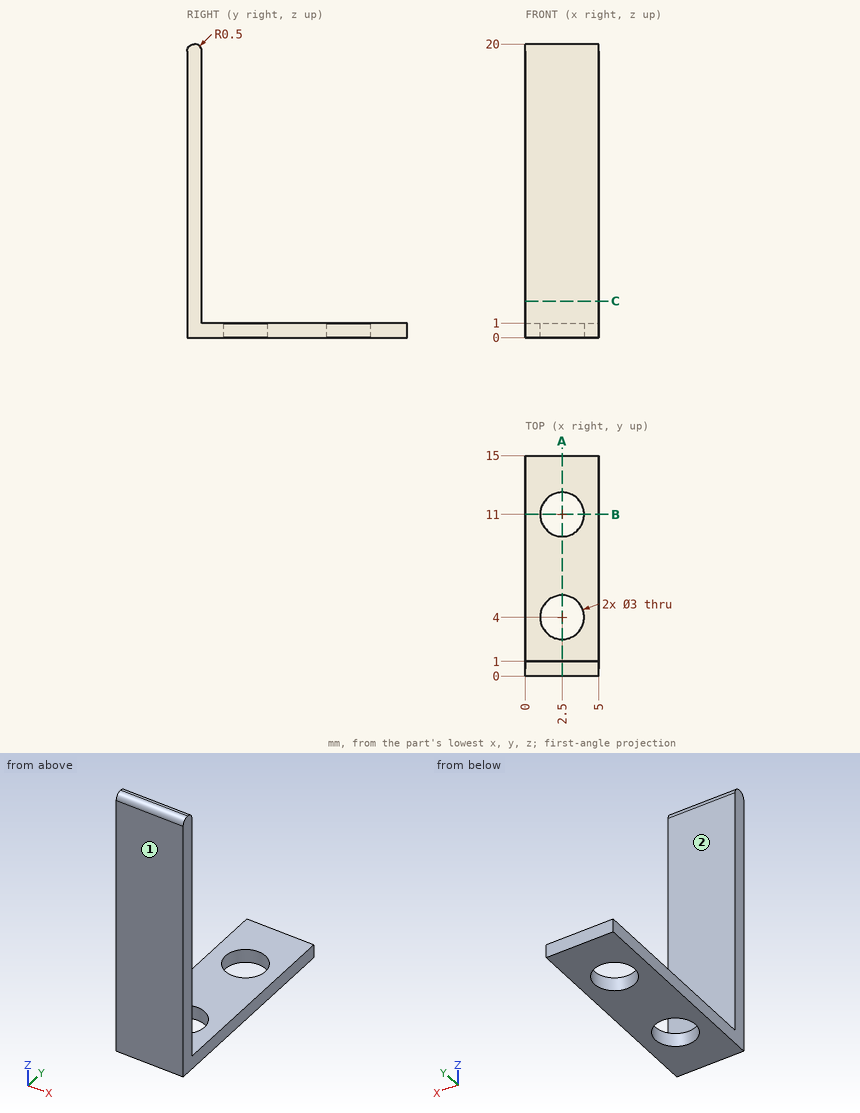
Answer from the drawing. Dimensions are ordinates in mm from the lowest x, y and z of the part. A direction names the side the tool comes from. Round coordinates to 2 decimals unless told otherwise and drop trailing zeros. Loops run counter-clockwise (first coordinate to the right, second up) from the corner with the lowest first, then second, coordinate; pieces in that order, holes last. Notation, with made-up numbers: (41.25, 84) - (99.25, 84) arc R27 cw to (99.25, 119) - close; hole circle Ø10 at (-8.75, -33.75). An arc over 180 degrees is marked (long way). One line per item, written item: value.
Q1. Find section A-A on x = 2.5. State how many separate pieces and enclosed holes the cut face has, and give its area (3 significant figures).
Check values:
separate pieces: 3
enclosed holes: 0
area: 27.9 mm2
Q2. Straight lines are drawn through the part: probe 1 along Y at (x, z) = (2.5, 0.25); probe 2 along Z at (x, y) = (1.45, 13.75). For each, find the intervals that lie inside material, in ascending order.
Check values:
probe 1: 0 to 2.5, 5.5 to 9.5, 12.5 to 15
probe 2: 0 to 1
Q3. Find section B-B on y = 11. Give the vertices of the cut face in (x, z), and give its area (3 significant figures).
Check values:
outline: (0, 0) - (1, 0) - (1, 1) - (0, 1) - close; (4, 0) - (5, 0) - (5, 1) - (4, 1) - close
area: 2.00 mm2
Q4. Find section C-C on z = 2.5. Give the vertices of the cut face in (x, y).
Check values:
outline: (0, 0) - (5, 0) - (5, 1) - (0, 1) - close
Q5. For the marked faces 1 and 2, determine the directions among +Z, -Z, +X, -X, +Y, -Y from which every point of the face is accessible in a straight line to the end or side of a thin tool.
Check values:
face 1: +Z, -Z, +X, -X, -Y
face 2: +Z, +X, -X, +Y
Q6. Each of these flat-tipped pins is pushed along its axis until it touches: pin 1 Ø3 at (x, z) = (1.5, 4) entering from +Y; pin 2 Ø1.5 at (x, y) = (1, 3) entering from +Z. Where does it stop, or does it pass through?
Check values:
pin 1: y = 1
pin 2: z = 1
